```python
from build123d import *

# Parameters (mm, degrees)
F0_R     = 2.5
F1_DEPTH = 15


# Not quite as in the source:
# - a fillet or chamfer that OpenCascade refuses, or shapes differently, is made with other operations: its cross-section is extruded or revolved along the edge and cut away or added


with BuildPart() as f1:
    # F0 (on Top) → F1 (new body)
    with BuildSketch(Plane.XY):
        Polygon((-7.5, 10), (-17.5, 10), (-17.5, 5), (-17.5, -10), (17.5, -10), (17.5, 10), align=None)
        with Locations((-12.5, -5)):
            Circle(F0_R, mode=Mode.SUBTRACT)
        with Locations((12.5, -5)):
            Circle(F0_R, mode=Mode.SUBTRACT)
        with BuildLine():
            ThreePointArc((-10, 5), (-12.5, 2.5), (-15, 5))
            ThreePointArc((-15, 5), (-12.5, 7.5), (-10, 5))
        make_face(mode=Mode.SUBTRACT)
        Circle(F0_R, mode=Mode.SUBTRACT)
        with Locations((12.5, 5)):
            Circle(F0_R, mode=Mode.SUBTRACT)
    extrude(amount=F1_DEPTH)

    # F2: chamfer of 3 on 5 edges, made by hand

    # F2_s1 → F2_t2 (revolve, cut)
    with BuildSketch(Plane.XZ.offset(-5)):
        Polygon((-7, 15), (-10, 12), (-10, 15), align=None)
    revolve(axis=Axis((-12.5, 5, 15), (0, 0, 1)), mode=Mode.SUBTRACT)

    # F2_s3 → F2_t4 (revolve, cut)
    with BuildSketch(Plane.XZ):
        Polygon((5.5, 15), (2.5, 12), (2.5, 15), align=None)
    revolve(axis=Axis((0, 0, 15), (0, 0, 1)), mode=Mode.SUBTRACT)

    # F2_s5 → F2_t6 (revolve, cut)
    with BuildSketch(Plane.XZ.offset(5)):
        Polygon((-7, 15), (-10, 12), (-10, 15), align=None)
    revolve(axis=Axis((-12.5, -5, 15), (0, 0, 1)), mode=Mode.SUBTRACT)

    # F2_s7 → F2_t8 (revolve, cut)
    with BuildSketch(Plane.XZ.offset(-5)):
        Polygon((18, 15), (15, 12), (15, 15), align=None)
    revolve(axis=Axis((12.5, 5, 15), (0, 0, 1)), mode=Mode.SUBTRACT)

    # F2_s9 → F2_t10 (revolve, cut)
    with BuildSketch(Plane.XZ.offset(5)):
        Polygon((18, 15), (15, 12), (15, 15), align=None)
    revolve(axis=Axis((12.5, -5, 15), (0, 0, 1)), mode=Mode.SUBTRACT)


solid = f1.part
```
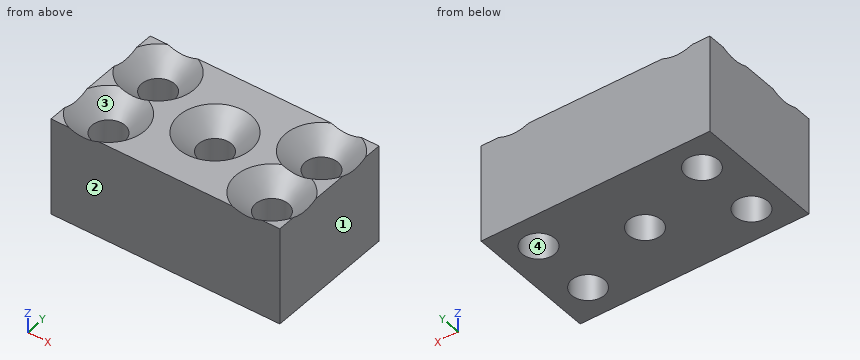
The listing builds one solid part. Answer for the finished solid, in the listing's coordinates (mm). Face numbers are marked on the shaded views. Coordinates: 2 decimals unless noted, no trailing zeros. Loops run counter-clockwise (first coordinate to the right, second up) from the corner with the lowest first, then second, coordinate; pieces in that order, holes last. Notation, with made-up numbers: M 48,1 L 92,1 A20 cw 92,17 Z; hole C 9.5,-20.75 d8. An arc over 180 degrees is marked long. Answer as a JSON object with one key per item and string values. Group by question number.
Item 1: Section B-B (x = 12.5) is taken. Write down the section's boundary in (y, z).
Item 2: Consider L1, parallel to Y at x = -12.5, z = 5.75; L2, parallel to Y at x = 0, z = 4.25; L3, parallel to X at y = -6.75, z = 5. Determine where each line is inside the solid, lowest interval first.
Item 3: Section D-D (y = 3.25) is taken. Give the number of separate pieces and of enclosed holes in the cut face, and give its area (3 significant figures).
Item 4: Determine the mould class of the marked faces 1, 2, 3 and 4 for opening direction Y: +Y half, -Y half, draft (parallel to the pull), parting line (faces both ways), or undercut.
Item 5: This flat-tipped pin is pushed along its axis until it touches: P1, Ø8, axis at x = 0, y = 0, coming from the +Z side. Where does it stop, or does it pass through?
Item 6: Section A-A (x = 0) is taken. Write down the section's boundary in (y, z), and give its area (3 significant figures).
Item 7: Section C-C (z = 1) is taken. Write down the section's boundary in (x, y).
Solved:
{
 "1": {"outline": "M -10,0 L -7.5,0 L -7.5,12 L -10,14.5 Z; M -2.5,0 L 2.5,0 L 2.5,12 L 0,14.5 L -2.5,12 Z; M 7.5,0 L 10,0 L 10,14.5 L 7.5,12 Z"},
 "2": {"L1": "y = -10 to -7.5, -2.5 to 2.5, 7.5 to 10", "L2": "y = -10 to -2.5, 2.5 to 10", "L3": "x = -17.5 to -14.29, -10.71 to 10.71, 14.29 to 17.5"},
 "3": {"separate pieces": "3", "enclosed holes": "0", "area": "384 mm2"},
 "4": {"face 1": "draft", "face 2": "-Y half", "face 3": "undercut", "face 4": "undercut"},
 "5": {"P1": "stops at z = 13.5"},
 "6": {"outline": "M -10,0 L -2.5,0 L -2.5,12 L -5.5,15 L -10,15 Z; M 2.5,0 L 10,0 L 10,15 L 5.5,15 L 2.5,12 Z", "area": "216 mm2"},
 "7": {"outline": "M -17.5,-10 L 17.5,-10 L 17.5,10 L -17.5,10 Z; hole C -12.5,-5 d5; hole C -12.5,5 d5; hole C 0,0 d5; hole C 12.5,-5 d5; hole C 12.5,5 d5"}
}
